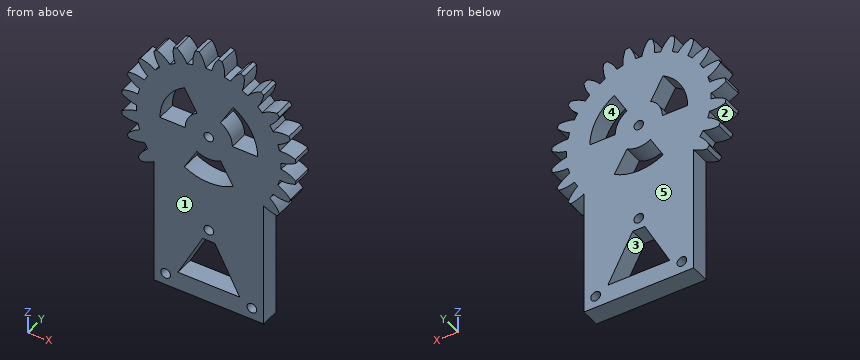
from build123d import *

# Parameters (mm, degrees)
SKETCH1_R           = 1.4
SKETCH1_R_2         = 1.44
BOSS_EXTRUDE2_DEPTH = 5.7


with BuildPart() as part:
    # Sketch1 → Boss-Extrude2 (new body)
    with BuildSketch(Plane(origin=(0, 0, 0), x_dir=(1, 0, 0), z_dir=(0, 1, 0))):
        with BuildLine():
            Line((16.282643734, -55.473929669), (-16.294749294, -55.473929669))
            Line((-16.294749294, -55.473929669), (-16.294749294, -92.997636196))
            ThreePointArc((-16.294749294, -92.997636196), (-18.191440049, -92.050885637), (-20.249670305, -91.543479832))
            ThreePointArc((-20.249670305, -91.543479832), (-20.602163218, -91.991288827), (-20.944755668, -92.446716717))
            ThreePointArc((-20.944755668, -92.446716717), (-19.764567011, -94.531247615), (-18.105041425, -96.258699254))
            ThreePointArc((-18.105041425, -96.258699254), (-18.601337045, -97.073436545), (-19.060996376, -97.909390787))
            ThreePointArc((-19.060996376, -97.909390787), (-21.385246964, -97.329758545), (-23.780643137, -97.343597276))
            ThreePointArc((-23.780643137, -97.343597276), (-24.005836083, -97.869056559), (-24.219420722, -98.399340372))
            ThreePointArc((-24.219420722, -98.399340372), (-22.53946113, -100.106926418), (-20.489045224, -101.345437195))
            ThreePointArc((-20.489045224, -101.345437195), (-20.758075202, -102.263784688), (-20.985968299, -103.193195246))
            ThreePointArc((-20.985968299, -103.193195246), (-23.3810186, -103.236188129), (-25.690864, -103.870797115))
            ThreePointArc((-25.690864, -103.870797115), (-25.775064405, -104.459357336), (-25.845783772, -105.049689119))
            ThreePointArc((-25.845783772, -105.049689119), (-23.779779823, -106.262018289), (-21.477950818, -106.92511524))
            ThreePointArc((-21.477950818, -106.92511524), (-21.497710797, -107.846662377), (-21.477950818, -108.768209514))
            ThreePointArc((-21.477950818, -108.768209514), (-23.780746321, -109.427942192), (-25.848519588, -110.637251105))
            ThreePointArc((-25.848519588, -110.637251105), (-25.781205181, -111.202699229), (-25.701523459, -111.766537533))
            ThreePointArc((-25.701523459, -111.766537533), (-23.393073925, -112.406205481), (-20.998123562, -112.454445414))
            ThreePointArc((-20.998123562, -112.454445414), (-20.773235617, -113.38074943), (-20.507508787, -114.296174451))
            ThreePointArc((-20.507508787, -114.296174451), (-22.561079267, -115.529447584), (-24.245391936, -117.232740033))
            ThreePointArc((-24.245391936, -117.232740033), (-24.033987825, -117.761573279), (-23.811051179, -118.285649183))
            ThreePointArc((-23.811051179, -118.285649183), (-21.415701651, -118.306020019), (-19.089879068, -117.732728078))
            ThreePointArc((-19.089879068, -117.732728078), (-18.6328306, -118.56937566), (-18.139140457, -119.384938363))
            ThreePointArc((-18.139140457, -119.384938363), (-19.803499131, -121.107733922), (-20.989523145, -123.188950243))
            ThreePointArc((-20.989523145, -123.188950243), (-20.6482393, -123.645300692), (-20.297036031, -124.094061943))
            ThreePointArc((-20.297036031, -124.094061943), (-17.978064026, -123.493659436), (-15.879929184, -122.337828774))
            ThreePointArc((-15.879929184, -122.337828774), (-15.221495643, -123.028026694), (-14.533094291, -123.688338344))
            ThreePointArc((-14.533094291, -123.688338344), (-15.694637363, -125.783316155), (-16.301356047, -128.100643661))
            ThreePointArc((-16.301356047, -128.100643661), (-15.852512396, -128.453869244), (-15.396017905, -128.797150052))
            ThreePointArc((-15.396017905, -128.797150052), (-13.311697063, -127.616590454), (-11.584540779, -125.95675748))
            ThreePointArc((-11.584540779, -125.95675748), (-10.767926313, -126.453945848), (-9.930014765, -126.914336658))
            ThreePointArc((-9.930014765, -126.914336658), (-10.50881973, -129.2387934), (-10.494128437, -131.634184496))
            ThreePointArc((-10.494128437, -131.634184496), (-9.96421413, -131.861006909), (-9.429401724, -132.076026145))
            ThreePointArc((-9.429401724, -132.076026145), (-7.723011964, -130.394851461), (-6.485961057, -128.34355446))
            ThreePointArc((-6.485961057, -128.34355446), (-5.571070397, -128.610954069), (-4.645226545, -128.837538785))
            ThreePointArc((-4.645226545, -128.837538785), (-4.607931078, -131.230595815), (-3.979841993, -133.540058306))
            ThreePointArc((-3.979841993, -133.540058306), (-3.404307437, -133.622657246), (-2.827069767, -133.692365802))
            ThreePointArc((-2.827069767, -133.692365802), (-1.614740596, -131.626361853), (-0.951643646, -129.324532848))
            ThreePointArc((-0.951643646, -129.324532848), (0.001289203, -129.345662377), (0.954222052, -129.324532848))
            ThreePointArc((0.954222052, -129.324532848), (1.605623598, -131.625984951), (2.805751963, -133.694969645))
            ThreePointArc((2.805751963, -133.694969645), (3.383053833, -133.62579479), (3.958664509, -133.543727981))
            ThreePointArc((3.958664509, -133.543727981), (4.594963395, -131.234347532), (4.63970868, -128.839329329))
            ThreePointArc((4.63970868, -128.839329329), (5.565639854, -128.613101716), (6.480633579, -128.346054989))
            ThreePointArc((6.480633579, -128.346054989), (7.716893233, -130.397828953), (9.422634458, -132.079661646))
            ThreePointArc((9.422634458, -132.079661646), (9.951058445, -131.867530222), (10.474710197, -131.643877606))
            ThreePointArc((10.474710197, -131.643877606), (10.491616082, -129.248501117), (9.914960384, -126.923510248))
            ThreePointArc((9.914960384, -126.923510248), (10.750789203, -126.465342533), (11.565488494, -125.9705774))
            ThreePointArc((11.565488494, -125.9705774), (13.290661801, -127.632471318), (15.373571634, -128.815518637))
            ThreePointArc((15.373571634, -128.815518637), (15.829086357, -128.473849224), (16.277009552, -128.12228634))
            ThreePointArc((16.277009552, -128.12228634), (15.673370328, -125.804154761), (14.514611779, -123.707635512))
            ThreePointArc((14.514611779, -123.707635512), (15.203377892, -123.048751065), (15.862262338, -122.359984953))
            ThreePointArc((15.862262338, -122.359984953), (17.958781587, -123.518743501), (20.276913167, -124.122382726))
            ThreePointArc((20.276913167, -124.122382726), (20.628476051, -123.674459531), (20.970145463, -123.218944808))
            ThreePointArc((20.970145463, -123.218944808), (19.787098144, -121.136034974), (18.125204226, -119.410861668))
            ThreePointArc((18.125204226, -119.410861668), (18.619969359, -118.596162377), (19.078137075, -117.760333557))
            ThreePointArc((19.078137075, -117.760333557), (21.403127944, -118.336989255), (23.798504433, -118.32008337))
            ThreePointArc((23.798504433, -118.32008337), (24.022157048, -117.796431618), (24.234288472, -117.268007632))
            ThreePointArc((24.234288472, -117.268007632), (22.552455779, -115.562266407), (20.500681815, -114.326006752))
            ThreePointArc((20.500681815, -114.326006752), (20.767728542, -113.411013027), (20.993956155, -112.485081853))
            ThreePointArc((20.993956155, -112.485081853), (23.388974358, -112.440336569), (25.698354808, -111.804037682))
            ThreePointArc((25.698354808, -111.804037682), (25.778855599, -111.240343374), (25.846992628, -110.675021347))
            ThreePointArc((25.846992628, -110.675021347), (23.780988679, -109.462692176), (21.479159674, -108.799595225))
            ThreePointArc((21.479159674, -108.799595225), (21.500289203, -107.846662377), (21.479159674, -106.893729528))
            ThreePointArc((21.479159674, -106.893729528), (23.780988679, -106.230632577), (25.846992628, -105.018303407))
            ThreePointArc((25.846992628, -105.018303407), (25.778855599, -104.452981379), (25.698354808, -103.889287071))
            ThreePointArc((25.698354808, -103.889287071), (23.388974358, -103.252988184), (20.993956155, -103.2082429))
            ThreePointArc((20.993956155, -103.2082429), (20.767728542, -102.282311726), (20.500681815, -101.367318001))
            ThreePointArc((20.500681815, -101.367318001), (22.552455779, -100.131058346), (24.234288472, -98.425317121))
            ThreePointArc((24.234288472, -98.425317121), (24.022157048, -97.896893135), (23.798504433, -97.373241383))
            ThreePointArc((23.798504433, -97.373241383), (21.403127944, -97.356335498), (19.078137075, -97.932991196))
            ThreePointArc((19.078137075, -97.932991196), (18.619969359, -97.097162377), (18.125204226, -96.282463086))
            ThreePointArc((18.125204226, -96.282463086), (19.787098144, -94.557289779), (20.970145463, -92.474379945))
            ThreePointArc((20.970145463, -92.474379945), (20.628476051, -92.018865222), (20.276913167, -91.570942027))
            ThreePointArc((20.276913167, -91.570942027), (18.197116907, -92.083089067), (16.282643734, -93.043630342))
            Line((16.282643734, -93.043630342), (16.282643734, -55.473929669))
        make_face()
        with BuildLine():
            ThreePointArc((-6.998710797, -107.846662377), (-6.060888623, -111.346662377), (-3.498710797, -113.908840203))
            Line((-3.498710797, -113.908840203), (-7.248210797, -120.403164706))
            ThreePointArc((-7.248210797, -120.403164706), (-12.555213127, -115.096162377), (-14.497710797, -107.846662377))
            Line((-14.497710797, -107.846662377), (-6.998710797, -107.846662377))
        make_face(mode=Mode.SUBTRACT)
        with Locations((0.001289203, -107.846662377)):
            Circle(SKETCH1_R, mode=Mode.SUBTRACT)
        with BuildLine():
            Line((7.250789203, -120.403164706), (3.501289203, -113.908840203))
            ThreePointArc((3.501289203, -113.908840203), (6.06346703, -111.346662377), (7.001289203, -107.846662377))
            Line((7.001289203, -107.846662377), (14.500289203, -107.846662377))
            ThreePointArc((14.500289203, -107.846662377), (12.557791533, -115.096162377), (7.250789203, -120.403164706))
        make_face(mode=Mode.SUBTRACT)
        with BuildLine():
            Line((7.250246793, -95.289846902), (3.501289203, -101.78448455))
            ThreePointArc((3.501289203, -101.78448455), (0.001289203, -100.846662377), (-3.498710797, -101.78448455))
            Line((-3.498710797, -101.78448455), (-7.248210797, -95.290160047))
            ThreePointArc((-7.248210797, -95.290160047), (0.000976046, -93.34766238), (7.250246793, -95.289846902))
        make_face(mode=Mode.SUBTRACT)
        with Locations((-12.8, -58.985750662)):
            Circle(SKETCH1_R_2, mode=Mode.SUBTRACT)
        with Locations((0, -78.242875331)):
            Circle(SKETCH1_R_2, mode=Mode.SUBTRACT)
        Polygon((-1.8, -74.867693206), (-9.18, -60.945750662), (9.18, -60.945750662), (1.8, -74.867693206), align=None, mode=Mode.SUBTRACT)
        with Locations((12.8, -58.985750662)):
            Circle(SKETCH1_R_2, mode=Mode.SUBTRACT)
    extrude(amount=BOSS_EXTRUDE2_DEPTH)


solid = part.part
CAD build for the part. Positions are in the model's coordinates, mm. Face numbers are marked on the shaded views. A direction names the side the tool comes from. Coordinates: 2 decimals unless noted, no trailing zeros. Order: outer loops, then holes, each group sorted by start corner. A loop starts at its lowest first (then second) coordinate and runs counter-clockwise, first axis right, second up. Notation, with made-up numbers: (-28.5, 22) -> (-11.5, 22) arc R17 cw to (-11.5, 45) -> close; hole circle Ø9 at (-13.75, 28.5). An arc over 180 degrees is marked (long way). Answer in a Markdown table with one row per item.
1) Which spindle directions (+Z, -Z, +X, -X, +Y, -Y) get a long thin tool onto all of the face, cutting with end or side? Do the marked faces 4 and 5. Say none if no direction does.
Check values:
| item | result |
|---|---|
| face 4 | +Y, -Y |
| face 5 | +Z, -Z, +X, -X, +Y |
2) Band-saw the part on D-D (x = -12.8). List the corners of the cut face in (y, z).
Check values:
| item | result |
|---|---|
| outline | (0, 55.47) -> (5.7, 55.47) -> (5.7, 57.55) -> (0, 57.55) -> close; (0, 60.43) -> (5.7, 60.43) -> (5.7, 107.85) -> (0, 107.85) -> close; (0, 114.65) -> (5.7, 114.65) -> (5.7, 127.21) -> (0, 127.21) -> close |
3) Band-saw the part on A-A (x = 0). List the corners of the cut face in (y, z).
Check values:
| item | result |
|---|---|
| outline | (0, 55.47) -> (5.7, 55.47) -> (5.7, 60.95) -> (0, 60.95) -> close; (0, 74.87) -> (5.7, 74.87) -> (5.7, 76.8) -> (0, 76.8) -> close; (0, 79.68) -> (5.7, 79.68) -> (5.7, 93.35) -> (0, 93.35) -> close; (0, 100.85) -> (5.7, 100.85) -> (5.7, 106.45) -> (0, 106.45) -> close; (0, 109.25) -> (5.7, 109.25) -> (5.7, 129.35) -> (0, 129.35) -> close |
4) Band-saw the part on B-B (x = 12.8). List the corners of the cut face in (y, z).
Check values:
| item | result |
|---|---|
| outline | (0, 55.47) -> (5.7, 55.47) -> (5.7, 57.55) -> (0, 57.55) -> close; (0, 60.43) -> (5.7, 60.43) -> (5.7, 107.85) -> (0, 107.85) -> close; (0, 114.66) -> (5.7, 114.66) -> (5.7, 127.24) -> (0, 127.24) -> close |
5) Mould opens along X. For the marked faces 1, 2 and 3 say: pulls with the +X half, pulls with the -X half, needs draft (parallel to the pull), parting line crosses it, or undercut.
Check values:
| item | result |
|---|---|
| face 1 | needs draft |
| face 2 | undercut |
| face 3 | undercut |
6) Flat gauge pins, fed straight in: P1, Ø4, axis at x = -19.5, z = 100.5, coming from the -Y side; P2, Ø1, axis at x = -8, y = 1, coming from the +Z side; P3, Ø2, axis at y = 4, z = 85.5, coming from the +X side; P4, Ø3, axis at y = 1.5, z = 78.5, coming from the -X side. Where does each tip first touch, or does it go through?
Check values:
| item | result |
|---|---|
| P1 | y = 0 |
| P2 | z = 131.27 |
| P3 | x = 16.28 |
| P4 | x = -16.29 |
7) Band-saw the part on C-C (y = 3.05). Give the number of separate pieces and of enclosed holes in the cut face, and give its area (3 significant figures).
Check values:
| item | result |
|---|---|
| separate pieces | 1 |
| enclosed holes | 8 |
| area | 2,330 mm2 |
8) Drill centre lines: line 1 (Z direction, x = 0, y = 1.8); line 2 (X direction, y = 2, z = 110); line 3 (X direction, y = 0.9, z = 128). Where is each one in solid material? Low to high.
Check values:
| item | result |
|---|---|
| line 1 | 55.47 to 60.95, 74.87 to 76.8, 79.68 to 93.35, 100.85 to 106.45, 109.25 to 129.35 |
| line 2 | -24.91 to -14.34, -6.66 to 6.66, 14.34 to 24.84 |
| line 3 | -16.29 to -13.87, -10.28 to 10.26, 13.82 to 16.26 |
